Source: three-view drawing plus pictorial views. Frame: mm from the lowest corner of the part. A direction names the side the tool comes from. Give positions to 0.01 mm unless a question says otherwise; leave off trailing zeros. Order: outer loops, then holes, each group sorted by start corner. A loop starts at its lowest first (then second) coordinate and runs counter-clockwise, first axis right, second up. Notation, with made-up numbers: (34, 37.25) -> (93, 37.25) arc R21 ccw to (93, 44.25) -> close; hole circle Ø10 at (-0.5, 34). An arc over 180 degrees is marked (long way). Answer in a Markdown table with one row per item.
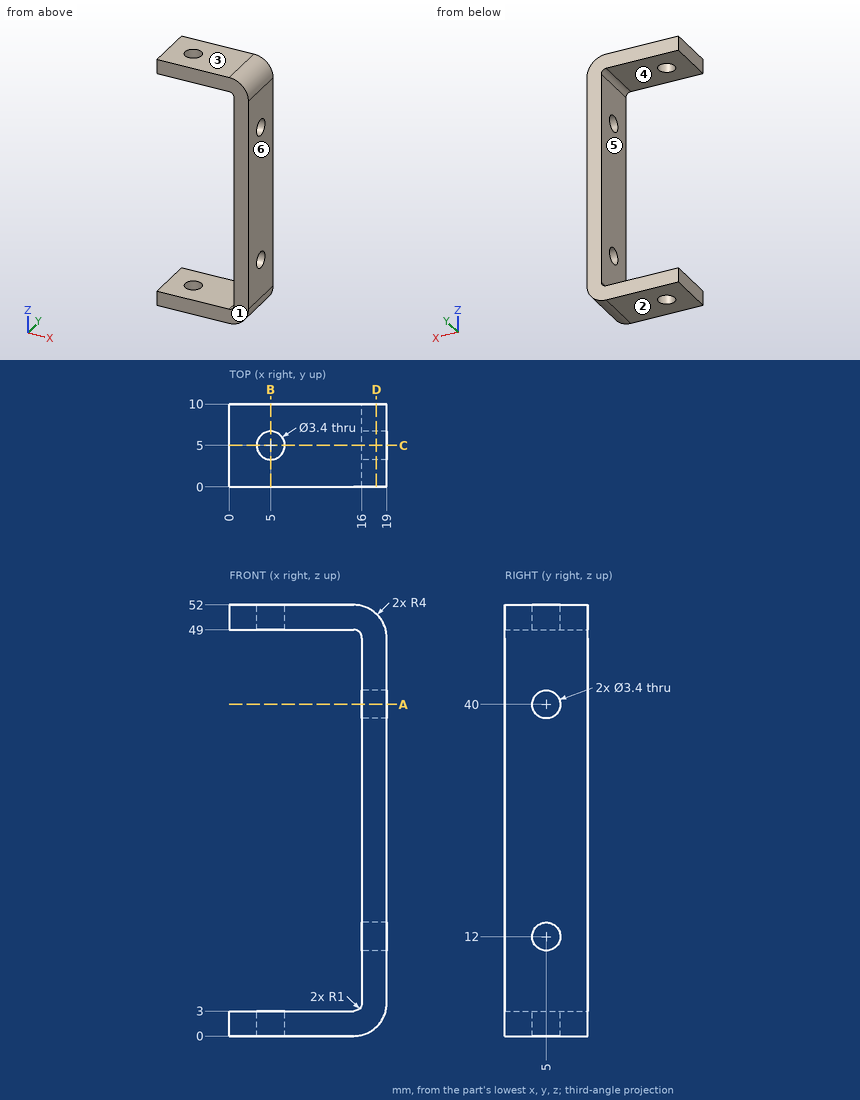
(1) Ray query, probe 1 along Z at (x, y) = (1.25, 2); probe 2 along Y at (x, z) = (17, 12); probe 3 along X at (y, z) = (6.75, 27.5). Return the intervals inside material, ascending.
A:
| item | result |
|---|---|
| probe 1 | z = 0 to 3, 49 to 52 |
| probe 2 | y = 0 to 3.3, 6.7 to 10 |
| probe 3 | x = 16 to 19 |
(2) Section query D-D (x = 17.75). Return the cut outline in (y, z).
A:
| item | result |
|---|---|
| outline | (0, 1.1) -> (10, 1.1) -> (10, 50.9) -> (0, 50.9) -> close; hole circle Ø3.4 at (5, 12); hole circle Ø3.4 at (5, 40) |
(3) Access query for the marked faces 5 and 6. Directions: +Z, -Z, +X, -X, +Y, -Y. A direction counts if a zero-diameter tool reaches every point of the face in a straight line with its end or side. Return the directions, or none.
A:
| item | result |
|---|---|
| face 5 | -X, +Y, -Y |
| face 6 | +Z, -Z, +X, +Y, -Y |
(4) First-contact query: pin 1 Ø2 at (y, z) = (5, 40) entering from -X; pin 2 Ø4 at (x, y) = (5, 5) entering from -Z. Flat tips, straight axial feed; report the tip coordinate or a pass-through.
A:
| item | result |
|---|---|
| pin 1 | passes through |
| pin 2 | stops at z = 0 |
(5) Section query C-C (y = 5). Return the cut outline in (x, z).
A:
| item | result |
|---|---|
| outline | (0, 0) -> (3.3, 0) -> (3.3, 3) -> (0, 3) -> close; (0, 49) -> (3.3, 49) -> (3.3, 52) -> (0, 52) -> close; (6.7, 0) -> (15, 0) arc R4 ccw to (19, 4) -> (19, 10.3) -> (16, 10.3) -> (16, 4) arc R1 cw to (15, 3) -> (6.7, 3) -> close; (6.7, 49) -> (15, 49) arc R1 cw to (16, 48) -> (16, 41.7) -> (19, 41.7) -> (19, 48) arc R4 ccw to (15, 52) -> (6.7, 52) -> close; (16, 13.7) -> (19, 13.7) -> (19, 38.3) -> (16, 38.3) -> close |
(6) Section query B-B (x = 5). Return the cut outline in (y, z), plus the area to 3 significant figures.
A:
| item | result |
|---|---|
| outline | (0, 0) -> (3.3, 0) -> (3.3, 3) -> (0, 3) -> close; (0, 49) -> (3.3, 49) -> (3.3, 52) -> (0, 52) -> close; (6.7, 0) -> (10, 0) -> (10, 3) -> (6.7, 3) -> close; (6.7, 49) -> (10, 49) -> (10, 52) -> (6.7, 52) -> close |
| area | 39.6 mm^2 |
(7) Pull-direction query (Z, two-part tool) for the marked faces 1, 2, 3 and 4; classes: +Z half, -Z half, draft (parallel to the pull), parting line (faces both ways), or undercut.
A:
| item | result |
|---|---|
| face 1 | draft |
| face 2 | -Z half |
| face 3 | +Z half |
| face 4 | undercut |
(8) Section query A-A (z = 40). Return the cut outline in (x, y), plus the area to 3 significant figures.
A:
| item | result |
|---|---|
| outline | (16, 0) -> (19, 0) -> (19, 3.3) -> (16, 3.3) -> close; (16, 6.7) -> (19, 6.7) -> (19, 10) -> (16, 10) -> close |
| area | 19.8 mm^2 |
